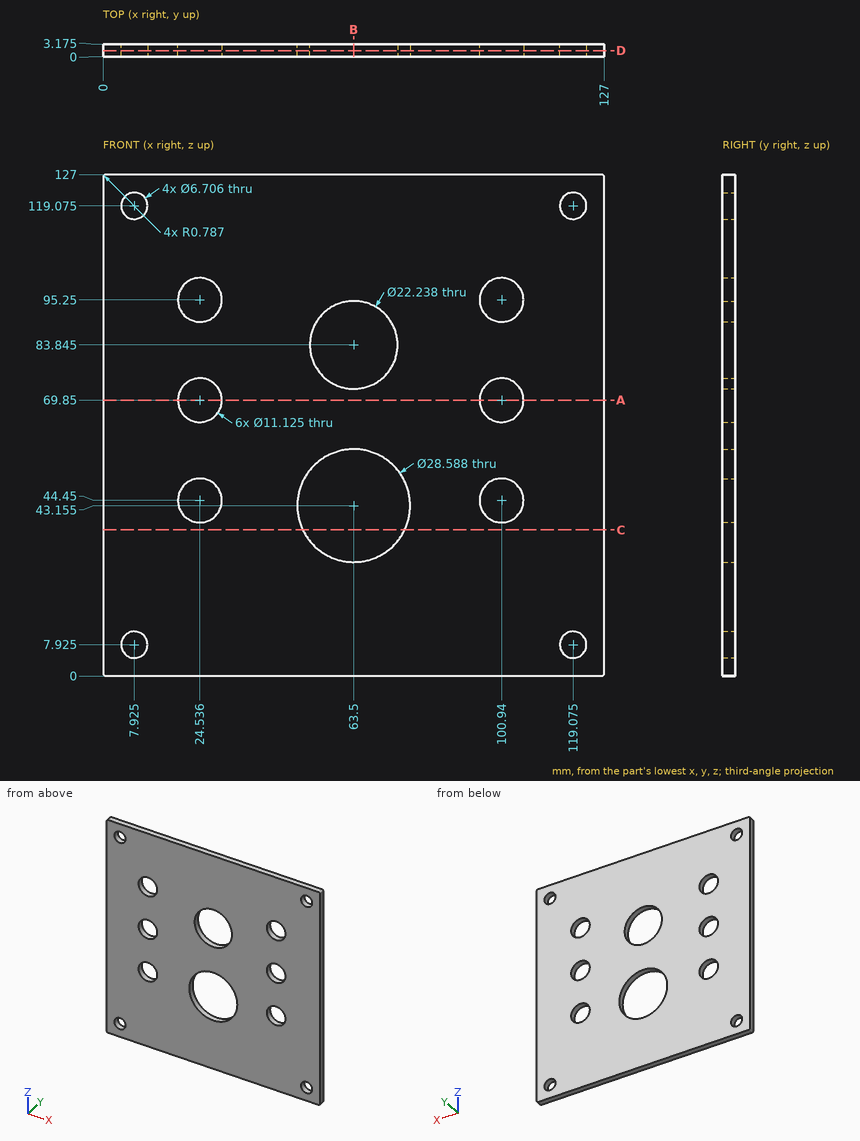
The figure shows three views and two pictorial views of one solid part (mm, origin at its lowest corner). Answer the questions. Round coordinates to 2 decimals unless told otherwise and drop trailing zeros. Write each loop counter-clockwise with the first axis right and the second up, starting at its lowest first coordinate (ties: lowest second). Pieces come first, ordered by that corner, then holes. Notation, with made-up numbers: (64.5, 7) -> (79.5, 7) arc R29 ccw to (79.5, 32) -> close; hole circle Ø5 at (79, -3). An arc over 180 degrees is marked (long way). Answer as a JSON object with one key per item and string values. Group by question number.
Q1. Section A-A (z = 69.85) is taken. Write down the section's boundary in (x, y) (1 decimal).
Q2. Section C-C (z = 37) is taken. Write down the section's boundary in (x, y) (1 decimal), plus the area to 3 significant figures.
Q3. Section B-B (x = 63.5) is taken. Write down the section's boundary in (y, z) (1 decimal), plus the area to 3 significant figures.
Q4. Section D-D (y = 1.5) is taken. Count the separate pieces of the cut face and the enclosed holes in it, plus the area to 3 significant figures.
Q5. Straight lines are drawn through the part: line 1 along Z through (x, y) = (24, 1.7); line 2 along X through (y, z) = (2.75, 119.5); line 3 along Z through (x, y) = (117.5, 3) (1 decimal). For each, find the intervals that lie inside material, in ascending order.
Q6. This flat-tipped pin is pushed along its axis until it touches: pin 1 Ø23 at (x, z) = (63.5, 43.15) entering from +Y. Where does it stop, or does it pass through?
Check values:
{
 "1": {"outline": "(0, 0) -> (19, 0) -> (19, 3.2) -> (0, 3.2) -> close; (30.1, 0) -> (95.4, 0) -> (95.4, 3.2) -> (30.1, 3.2) -> close; (106.5, 0) -> (127, 0) -> (127, 3.2) -> (106.5, 3.2) -> close"},
 "2": {"outline": "(0, 0) -> (50.6, 0) -> (50.6, 3.2) -> (0, 3.2) -> close; (76.4, 0) -> (127, 0) -> (127, 3.2) -> (76.4, 3.2) -> close", "area": "321 mm^2"},
 "3": {"outline": "(0, 0) -> (3.2, 0) -> (3.2, 28.9) -> (0, 28.9) -> close; (0, 57.4) -> (3.2, 57.4) -> (3.2, 72.7) -> (0, 72.7) -> close; (0, 95) -> (3.2, 95) -> (3.2, 127) -> (0, 127) -> close", "area": "242 mm^2"},
 "4": {"separate pieces": "1", "enclosed holes": "12", "area": "14,400 mm^2"},
 "5": {"line 1": "0 to 38.91, 49.99 to 64.31, 75.39 to 89.71, 100.79 to 127", "line 2": "0 to 4.6, 11.25 to 115.75, 122.4 to 127", "line 3": "0 to 5, 10.9 to 116.1, 122 to 127"},
 "6": {"pin 1": "through"}
}
